```python
from build123d import *
from build123d.topology import SkipClean

# Parameters (mm, degrees)
SKIZZE1_W                       = 200
SKIZZE1_H                       = 50
AUFSATZ_LINEAR_AUSTRAGEN1_DEPTH = 3
FASE1_SIZE                      = 25
AUFSATZ_LINEAR_AUSTRAGEN2_DEPTH = 11
SKIZZE3_W                       = 15.35533906
SKIZZE3_H                       = 11
SCHNITT_LINEAR_AUSTRAGEN1_DEPTH = 10
SKIZZE4_W                       = 15.35533906
SKIZZE4_H                       = 11
SCHNITT_LINEAR_AUSTRAGEN2_DEPTH = 10
SKIZZE5_W                       = 150
SKIZZE5_H                       = 12
AUFSATZ_LINEAR_AUSTRAGEN3_DEPTH = 5
AUFSATZ_LINEAR_AUSTRAGEN4_DEPTH = 11
AUFSATZ_LINEAR_AUSTRAGEN5_DEPTH = 11
SKIZZE12_R                      = 2.2
SCHNITT_LINEAR_AUSTRAGEN8_DEPTH = 10
AUFSATZ_LINEAR_AUSTRAGEN6_DEPTH = 11
SKIZZE8_R                       = 1.65
SKIZZE8_W                       = 3.016289267
SKIZZE8_H                       = 4
SCHNITT_LINEAR_AUSTRAGEN9_DEPTH = 10
AUFSATZ_LINEAR_AUSTRAGEN7_DEPTH = 1
SKIZZE11_R                      = 1.65
SKIZZE11_W                      = 2.95533906
SKIZZE11_H                      = 4
SCHNITT_LINEAR_AUSTRAGEN7_DEPTH = 10


with BuildPart() as part:
    # Skizze1 → Aufsatz-Linear austragen1 (new body)
    with BuildSketch(Plane(origin=(0, 0, 0), x_dir=(1, 0, 0), z_dir=(0, 1, 0))):
        Rectangle(SKIZZE1_W, SKIZZE1_H)
    extrude(amount=AUFSATZ_LINEAR_AUSTRAGEN1_DEPTH)

    # Fase1
    fase1_edges = [part.edges().sort_by_distance(p)[0] for p in [
        (-100, 1.5, -25),
        (-100, 1.5, 25),
        (100, 1.5, -25),
        (100, 1.5, 25),
    ]]
    chamfer(fase1_edges, length=FASE1_SIZE - 0.0001)  # a hair under: the kernel refuses the full size

    # Skizze2 → Aufsatz-Linear austragen2 (add)
    with BuildSketch(Plane(origin=(0, 3, 0), x_dir=(1, 0, 0), z_dir=(0, 1, 0))):
        Polygon((-73.177460326, 20.6), (-93.777460326, 0), (-73.277460326, -20.5), (73.277460326, -20.5), (93.777460326, 0), (73.177460326, 20.6), align=None)
        Polygon((90.949033201, 0), (72.349033201, 18.6), (-72.349033201, 18.6), (-90.949033201, 0), (-72.449033201, -18.5), (72.449033201, -18.5), align=None, mode=Mode.SUBTRACT)
    extrude(amount=AUFSATZ_LINEAR_AUSTRAGEN2_DEPTH)

    # Skizze3 → Schnitt-Linear austragen1 (cut)
    with BuildSketch(Plane(origin=(-46.888730163, 0, 46.888730163), x_dir=(0.7071067811865476, 0, 0.7071067811865476), z_dir=(-0.7071067811865476, 0, 0.7071067811865476))):
        with Locations((-53.033008589, 8.5)):
            Rectangle(SKIZZE3_W, SKIZZE3_H)
    extrude(amount=-SCHNITT_LINEAR_AUSTRAGEN1_DEPTH, mode=Mode.SUBTRACT)

    # Skizze4 → Schnitt-Linear austragen2 (cut)
    with BuildSketch(Plane(origin=(46.888730163, 0, 46.888730163), x_dir=(0.7071067811865475, 0, -0.7071067811865477), z_dir=(0.7071067811865477, 0, 0.7071067811865475))):
        with Locations((53.033008589, 8.5)):
            Rectangle(SKIZZE4_W, SKIZZE4_H)
    extrude(amount=-SCHNITT_LINEAR_AUSTRAGEN2_DEPTH, mode=Mode.SUBTRACT)

    # Skizze5 → Aufsatz-Linear austragen3 (add)
    with BuildSketch(Plane(origin=(0, 3, 0), x_dir=(1, 0, 0), z_dir=(0, 1, 0))):
        with Locations((-0.006490323, 0)):
            Rectangle(SKIZZE5_W, SKIZZE5_H)
    extrude(amount=AUFSATZ_LINEAR_AUSTRAGEN3_DEPTH)

    # Skizze6 → Aufsatz-Linear austragen4 (add)
    with BuildSketch(Plane(origin=(0, 3, 0), x_dir=(1, 0, 0), z_dir=(0, 1, 0))):
        Polygon((87.696342007, -3.252691193), (78.252691193, -12.696342007), (82.735076288, -17.264923712), (92.221825407, -7.778174593), align=None)
    extrude(amount=AUFSATZ_LINEAR_AUSTRAGEN4_DEPTH)

    # Skizze10 → Aufsatz-Linear austragen5 (add)
    with BuildSketch(Plane(origin=(0, 3, 0), x_dir=(1, 0, 0), z_dir=(0, 1, 0))):
        Polygon((-87.696342007, -3.252691193), (-78.252691193, -12.696342007), (-82.778174593, -17.221825407), (-92.221825407, -7.778174593), align=None)
    extrude(amount=AUFSATZ_LINEAR_AUSTRAGEN5_DEPTH)

    # Skizze12 → Schnitt-Linear austragen8 (cut)
    with BuildSketch(Plane(origin=(0, 3, 0), x_dir=(1, 0, 0), z_dir=(0, 1, 0))):
        with Locations(Location((0, 12.5, 0), (0, 0, 270))):
            Circle(SKIZZE12_R)
        with Locations(Location((0, -12.5, 0), (0, 0, 270))):
            Circle(SKIZZE12_R)
    extrude(amount=-SCHNITT_LINEAR_AUSTRAGEN8_DEPTH, mode=Mode.SUBTRACT)

    # Skizze13 → Aufsatz-Linear austragen6 (add)
    with BuildSketch(Plane(origin=(0, 3, 0), x_dir=(1, 0, 0), z_dir=(0, 1, 0))):
        Polygon((89.817662351, -3.959797975), (88.403448789, -2.545584412), (87.69285367, -3.256179531), (89.107067232, -4.670393094), align=None)
        Polygon((-89.817662351, -3.959797975), (-88.403448789, -2.545584412), (-87.689553601, -3.2594796), (-89.103767163, -4.673693162), align=None)
        Polygon((78.959797975, -14.817662351), (77.545584412, -13.403448789), (78.257117259, -12.691915942), (79.671330821, -14.106129505), align=None)
        Polygon((-78.959797975, -14.817662351), (-77.545584412, -13.403448789), (-78.262212477, -12.686820723), (-79.67642604, -14.101034286), align=None)
    extrude(amount=AUFSATZ_LINEAR_AUSTRAGEN6_DEPTH)

    # Skizze8 → Schnitt-Linear austragen9 (cut)
    with BuildSketch(Plane(origin=(50, 0, 50), x_dir=(0.7071067811865488, 0, -0.7071067811865465), z_dir=(0.7071067811865465, 0, 0.7071067811865488))):
        with Locations((49.294388852, 9)):
            Circle(SKIZZE8_R)
        with Locations((56.710678119, 9)):
            Circle(SKIZZE8_R)
        with Locations((53.002533486, 6)):
            Rectangle(SKIZZE8_W, SKIZZE8_H)
    extrude(amount=-SCHNITT_LINEAR_AUSTRAGEN9_DEPTH, mode=Mode.SUBTRACT)

    # Skizze14 → Aufsatz-Linear austragen7 (add)
    with SkipClean():  # the faces are left unmerged after this step: merging them gives an invalid solid
        with BuildSketch(Plane(origin=(0, 3, 0), x_dir=(1, 0, 0), z_dir=(0, 1, 0))):
            Polygon((-89.11055557, -4.666904756), (-93.777460326, 0), (-73.177460326, 20.6), (73.177460326, 20.6), (93.777460326, 0), (89.11055557, -4.666904756), (92.221825407, -7.778174593), (100, 0), (75, 25), (-75, 25), (-100, 0), (-92.221825407, -7.778174593), align=None)
            Polygon((-82.778174593, -17.221825407), (-79.666904756, -14.11055557), (-73.277460326, -20.5), (73.277460326, -20.5), (79.653436535, -14.12402379), (82.735076288, -17.264923712), (75, -25), (-75, -25), align=None)
        extrude(amount=AUFSATZ_LINEAR_AUSTRAGEN7_DEPTH)

    # Skizze11 → Schnitt-Linear austragen7 (cut)
    with SkipClean():  # the faces are left unmerged after this step: merging them gives an invalid solid
        with BuildSketch(Plane(origin=(-50, 0, 50), x_dir=(0.7071067811865465, 0, 0.7071067811865488), z_dir=(-0.7071067811865488, 0, 0.7071067811865465))):
            with Locations((-56.710678119, 9)):
                Circle(SKIZZE11_R)
            with Locations((-49.355339059, 9)):
                Circle(SKIZZE11_R)
            with Locations((-53.033008589, 6)):
                Rectangle(SKIZZE11_W, SKIZZE11_H)
        extrude(amount=-SCHNITT_LINEAR_AUSTRAGEN7_DEPTH, mode=Mode.SUBTRACT)


solid = part.part
```
Here's how the part is built. I have some questions about the finished solid (model axes, mm). A direction names the side the tool comes from. Give positions to 0.01 mm unless a question says otherwise; leave off trailing zeros. Loops run counter-clockwise (first coordinate to the right, second up) from the corner with the lowest first, then second, coordinate; pieces in that order, holes last. Notation, with made-up numbers: (-18.75, 30) -> (40.25, 30) arc R23 cw to (40.25, 58) -> close; hole circle Ø7 at (-21.5, 76.5). An arc over 180 degrees is marked (long way). Use one line per item in the form item = value. Start each with the question number.
1) Which directions (+Z, -Z, +X, -X, +Y, -Y) give clear straight access to the entire face, cutting with the end or side of a thin tool? Please do faces 5 (the face through (-1, 5, 6)), 6 (the face through (-84.22, 5.97, 11.31)), 7 (the face through (-90.688, 8.93, 6.244)).
2) For P1, Ø3, axis at x = 1.5, z = 18.5, coming from the -Y side; P2, Ø1, axis at y = 9, z = -19.5, coming from the +X side; P3, Ø4, axis at y = 4.5, z = 2, coming from the +X side; P4, Ø1, axis at x = 36.5, y = 6.5, coming from the -Z side, each with a flat end and sliding along its axis, tell me the tip position at first contact or that it passes through.
3) Please list where these lines run through material, in increasing order: line 1 along Z through (x, y) = (-16, 6.75); line 2 along Z through (x, y) = (8, 3.75); line 3 along Z through (x, y) = (58, 10.5).
4) Imagine slicing it at B-B (z = -12.5). Please give me the cut outline in (x, y).
5) Imagine slicing it at A-A (x = 0). Please give me the cut outline in (y, z), then the cut area to 4 significant figures.
6) Imagine slicing it at C-C (x = -65.5). Please give me the cut outline in (y, z).
7) Thinking about a two-plate mould opening in Y: for faces 1 (the face through (-88.8, 8, 6.74)), 2 (the face through (-85, 4, 10)), 3 (the face through (-1, 0, 0)), 4 (the face through (-81.201, 8.93, 15.644)), which applies, +Y half, -Y half, draft (parallel to the pull), parting line (faces both ways), or undercut?
8) Imagine slicing it at D-D (z = -3.5). Please give me the cut outline in (x, y), then the cut area to 3 significant figures.
Check values:
q1.face_5 = +Y
q1.face_6 = none
q1.face_7 = -X, +Y
q2.P1 = 0
q2.P2 = 74.78
q2.P3 = 99.94
q2.P4 = -20.6
q3.line_1 = -20.6 to -18.6, -6 to 6, 18.5 to 20.5
q3.line_2 = -25 to -18.6, -6 to 6, 18.5 to 25
q3.line_3 = -20.6 to -18.6, 18.5 to 20.5
q4.outline = (-87.5, 0) -> (-2.2, 0) -> (-2.2, 3) -> (-78.45, 3) -> (-78.45, 14) -> (-81.28, 14) -> (-81.28, 4) -> (-87.5, 4) -> close; (2.2, 0) -> (87.5, 0) -> (87.5, 4) -> (81.28, 4) -> (81.28, 14) -> (78.45, 14) -> (78.45, 3) -> (2.2, 3) -> close
q5.outline = (0, -25) -> (4, -25) -> (4, -20.6) -> (14, -20.6) -> (14, -18.6) -> (3, -18.6) -> (3, -14.7) -> (0, -14.7) -> close; (0, -10.3) -> (3, -10.3) -> (3, -6) -> (8, -6) -> (8, 6) -> (3, 6) -> (3, 10.3) -> (0, 10.3) -> close; (0, 14.7) -> (3, 14.7) -> (3, 18.5) -> (14, 18.5) -> (14, 20.5) -> (4, 20.5) -> (4, 25) -> (0, 25) -> close
q5.area = 236.5 mm^2
q6.outline = (0, -25) -> (4, -25) -> (4, -20.6) -> (14, -20.6) -> (14, -18.6) -> (3, -18.6) -> (3, -6) -> (8, -6) -> (8, 6) -> (3, 6) -> (3, 18.5) -> (14, 18.5) -> (14, 20.5) -> (4, 20.5) -> (4, 25) -> (0, 25) -> close
q7.face_1 = undercut
q7.face_2 = undercut
q7.face_3 = -Y half
q7.face_4 = draft
q8.outline = (-96.5, 0) -> (96.5, 0) -> (96.5, 4) -> (90.28, 4) -> (90.28, 14) -> (87.45, 14) -> (87.45, 3) -> (74.99, 3) -> (74.99, 8) -> (-75.01, 8) -> (-75.01, 3) -> (-87.45, 3) -> (-87.45, 14) -> (-90.28, 14) -> (-90.28, 4) -> (-96.5, 4) -> close
q8.area = 1,400 mm^2
